The listing builds one solid part. Answer for the finished solid, in the listing's coordinates (mm). A direction names the side the tool comes from. Coordinates: 2 decimals unless noted, no trailing zeros. Write each loop counter-clockwise with the first axis right and the second up, starting at its lowest first coordinate (ties: lowest second). Pieces come first, ordered by that corner, then holes.
from build123d import *

# Parameters (mm, degrees)
F1_DEPTH = 19.77278
F2_DEPTH = 15.68583
F3_DEPTH = 18.63252


with BuildPart() as f1:
    # F0 (on Right) → F1 (new body)
    with BuildSketch(Plane.YZ):
        with BuildLine():
            ThreePointArc((-24.6550113916, -20.6403282086), (-14.2899358418, -2.9499328055), (-21.631764082, 16.1937982509))
            ThreePointArc((-21.631764082, 16.1937982509), (-42.3952279546, 22.2110941878), (-59.3834631145, 8.8421320543))
            Line((-59.3834631145, 8.8421320543), (-28.7830121815, 8.8421320543))
            Line((-28.7830121815, 8.8421320543), (-20.9254194051, 0))
            Line((-20.9254194051, 0), (-28.4993667156, -10.8708310872))
            Line((-28.4993667156, -10.8708310872), (-59.3834631145, -10.8708310872))
            ThreePointArc((-59.3834631145, -10.8708310872), (-44.2799639395, -23.7919746243), (-24.6550113916, -20.6403282086))
        make_face()
    extrude(amount=F1_DEPTH)

    # F0 (on Right) → F2 (join)
    with BuildSketch(Plane.YZ):
        with BuildLine():
            ThreePointArc((77.5488621059, -18.7172400394), (70.5319981338, -6.4315126272), (76.3324780773, 6.4731342287))
            add(Edge.make_bspline(
                [(65.274477005, 3.5741054453), (66.7329266753, 3.4044171276), (70.0264053954, 3.0170299241), (74.0730411994, 5.2423594483), (76.3324780773, 6.4731342287)],
                knots=[0, 0, 0, 0, 0.4431105797, 1, 1, 1, 1], degree=3))
            Line((65.274477005, 3.5741054453), (-3.5807129461, 9.5008024946))
            add(Edge.make_bspline(
                [(-3.5807129461, 9.5008024946), (-8.1850167721, 10.4946023635), (-16.0626627691, 12.1809603216), (-19.9918558673, 15.0252283967), (-21.631764082, 16.1937982509)],
                knots=[0, 0, 0, 0, 0.5850187294, 1, 1, 1, 1], degree=3))
            ThreePointArc((-21.631764082, 16.1937982509), (-14.2899358418, -2.9499328055), (-24.6550113916, -20.6403282086))
            add(Edge.make_bspline(
                [(-5.0028073601, -17.0401390642), (-9.3359102028, -17.2862450952), (-17.1312640888, -17.7232079089), (-22.3392021757, -19.7477540646), (-24.6550113916, -20.6403282086)],
                knots=[0, 0, 0, 0, 0.5559843151, 1, 1, 1, 1], degree=3))
            Line((-5.0028073601, -17.0401390642), (65.274477005, -17.0401390642))
            add(Edge.make_bspline(
                [(65.274477005, -17.0401390642), (67.2859868291, -16.906336394), (71.3774576279, -16.6405736864), (75.4718135628, -18.0105027903), (77.5488621059, -18.7172400394)],
                knots=[0, 0, 0, 0, 0.4914160588, 1, 1, 1, 1], degree=3))
        make_face()
        with BuildLine():
            ThreePointArc((58.8446073234, 0), (65.572685649, -6.1609610629), (58.4222972393, -11.8263317272))
            Line((58.4222972393, -11.8263317272), (10.7007976621, -11.8263317272))
            ThreePointArc((10.7007976621, -11.8263317272), (1.6295820492, -4.0135137585), (10.365163526, 4.1728586721))
            Line((10.365163526, 4.1728586721), (58.8446073234, 0))
        make_face(mode=Mode.SUBTRACT)
    extrude(amount=F2_DEPTH)

    # F0 (on Right) → F3 (join)
    with BuildSketch(Plane.YZ):
        with BuildLine():
            Line((85.8887135983, 3.4065102227), (98.7935736775, 3.4065102227))
            ThreePointArc((98.7935736775, 3.4065102227), (88.2234276148, 9.7768503479), (76.3324780773, 6.4731342287))
            ThreePointArc((76.3324780773, 6.4731342287), (70.5319981338, -6.4315126272), (77.5488621059, -18.7172400394))
            ThreePointArc((77.5488621059, -18.7172400394), (89.1096263343, -20.9880157606), (98.9611595869, -14.5262060687))
            Line((98.9611595869, -14.5262060687), (87.73227036, -14.5262060687))
            Line((87.73227036, -14.5262060687), (80.8608531952, -4.6380725689))
            Line((80.8608531952, -4.6380725689), (85.8887135983, 3.4065102227))
        make_face()
    extrude(amount=F3_DEPTH)


solid = f1.part
Q1. Given pin 1 (2 mm diameter, centred on y = 30, z = 9, fed in from +X); pin 2 (8 mm diameter, centred on x = 11.5, y = 33.5, fed in from -Z); pin 3 (3 mm diameter, centred on x = 8.5, z = -16, fed in from -Y); pin 4 (10.5 mm diameter, centred on x = 5, y = 93.5, fed in from -Z), each flat-ended and moving along its own axis, determine where each tip first touches the part or whether it passes through.
Answers below:
pin 1: passes through
pin 2: stops at z = -17.04
pin 3: stops at y = -57.31
pin 4: stops at z = -21.13
Q2. Determine the mould class of faces 4 (the face through (7.7, 31.3, 6.5)), 5 (the face through (9, 92, 3.407)), 6 (the face through (8, 30, -17.04)) for opening direction Z: released by +Z, released by -Z, zero draft, split by the parting line, or undercut.
Answers below:
face 4: released by +Z
face 5: undercut
face 6: released by -Z
Q3. Which of the six approach directions +Z, -Z, +X, -X, +Y, -Y give full straight-line access (tool end or side, diameter ignored) to faces 1 (the face through (9.75, -24.66, -5.36)), 2 (the face through (8, 35, -11.826)), 3 (the face through (9.19, 83.34, -0.67))?
Answers below:
face 1: +X, -X, -Y
face 2: +X, -X
face 3: +X, -X, +Y
Q4. The part is cut by section A-A, the plane z = 1.5. Write down the section's boundary in (x, y).
Answers below:
outline: (0, -22.26) - (19.77, -22.26) - (19.77, -14.34) - (15.69, -14.34) - (15.69, 3.66) - (0, 3.66) - close; (0, 41.42) - (15.69, 41.42) - (15.69, 72.26) - (18.63, 72.26) - (18.63, 84.7) - (0, 84.7) - close
Q5. The part is cut by section D-D, the plane y = 30. Write down the section's boundary in (x, z).
Answers below:
outline: (0, -17.04) - (15.69, -17.04) - (15.69, -11.83) - (0, -11.83) - close; (0, 2.48) - (15.69, 2.48) - (15.69, 6.61) - (0, 6.61) - close
Q6. The part is cut by section B-B, the plane y = 4. Write down the section's boundary in (x, z).
Answers below:
outline: (0, -17.04) - (15.69, -17.04) - (15.69, -9.55) - (0, -9.55) - close; (0, 1.86) - (15.69, 1.86) - (15.69, 8.85) - (0, 8.85) - close
Q7. Find the intervals of material crossed by probe 1 along Y at (x, z) = (17.5, -3.5); probe 2 along Z at (x, y) = (6.5, 68); probe 3 along X at (y, z) = (-14, 7.5), in increasing order.
Answers below:
probe 1: y = -23.36 to -14.34, 70.67 to 81.57
probe 2: z = -16.9 to 3.38
probe 3: x = 0 to 15.69
Q8. The part is cut by section C-C, the plane z = -6. Write down the section's boundary in (x, y).
Answers below:
outline: (0, -25.11) - (19.77, -25.11) - (19.77, -14.74) - (15.69, -14.74) - (15.69, 1.92) - (0, 1.92) - close; (0, 65.58) - (15.69, 65.58) - (15.69, 70.52) - (18.63, 70.52) - (18.63, 81.81) - (0, 81.81) - close
